Part model, mm, in its own coordinate system. A direction names the side the tool comes from. Round coordinates to 2 decimals unless told otherwise and drop trailing zeros. Loops run counter-clockwise (first coordinate to the right, second up) from the corner with the lowest first, then second, coordinate; pieces in that order, holes last.
(1) Probe probe 1 along X at (y, z) = (42, -6); probe 2 along Z at (x, y) = (13.5, 49); probe 3 along Y at (x, z) = (10, -10.5). List the from-to ranges inside material, lowest first.
(2) Cut at A-A on y = 47. List the corners of the cut face in (x, z), then the cut area to 3 significant figures.
(3) Tool access for faces 4 (the face through (0.57, 48.49, -0.6)), 5 (the face through (29.4, 48.49, -0.57)), 6 (the face through (15, 44, -25)), 7 (the face through (15, 48, 0)), 8 (the face through (15, 3, 14)): list every direction of +Z, -Z, +X, -X, +Y, -Y with a clear straight run to the whole face (end or side of a thin tool).
(4) Mould opens along X. For faces 1 (the face through (5, 44, -15)), 2 (the face through (0.6, 42.08, -29.43)), 3 (the face through (29.43, 42.08, -29.4)) say: +X half, -X half, draft (parallel to the pull), parting line (faces both ways), or undercut.
(5) Flat gauge pins, fed straight in: pin 1 (6 mm diameter, centred on x = 17.5, z = 28.5, fed in from -Y); pin 2 (6 mm diameter, centred on x = 11, y = 64, fed in from +Z); pin 3 (8 mm diameter, centred on x = 17.5, z = 14.5, fed in from +Y). Where does each tip first touch, or does it go through?
(6) Cut at D-D on y = 7.5. List the corners of the cut face in (x, z).
Autodesk Inventor part; units mm, degrees
ref_plane "YZ Plane" through (0, 0, 0) normal (1, 0, 0) x (0, 1, 0)
ref_plane "XZ Plane" through (0, 0, 0) normal (0, 1, 0) x (-1, 0, 0)
ref_plane "XY Plane" through (0, 0, 0) normal (0, 0, 1) x (1, 0, 0)
sketch "Sketch1" plane through (0, 0, 0) normal (1, 0, 0) x (0, 1, 0)
  line L0 (0, 0) -> (0, -30)
  line L1 (11, 0) -> (30, 0) construction
  line L2 (0, -30) -> (85, -30)
  line L3 (11, 0) -> (85, 0)
  line L4 (85, 0) -> (85, -30)
  line L5 (0, 0) -> (0, 14)
  line L6 (11, 0) -> (14, 0) construction
  line L7 (0, 14) -> (6, 14)
  line L8 (6, 14) -> (6, 34)
  line L9 (6, 34) -> (11, 34)
  line L10 (11, 34) -> (11, 0)
  dimension "d0" = 30
  dimension "d2" = 85
  dimension "d4" = 14
  dimension "d6" = 6
  dimension "d7" = 20
  dimension "d8" = 5
  dimension "d9" = 34
extrude "Extrusion1" add sketch "Sketch1" along normal blind 30
sketch "Sketch2" plane through (0, 85, 0) normal (0, 1, 0) x (1, 0, 0)
  line L0 (5, 5) -> (5, 25)
  line L1 (5, 5) -> (25, 5) construction
  line L2 (5, 25) -> (25, 25)
  line L3 (25, 25) -> (25, 5)
  line L4 (25, 5) -> (5, 5)
  point P0 (0, 0)
  dimension "d13" = 20
  dimension "d14" = 90
  dimension "d15" = 20
  dimension "d16" = 90
  dimension "d17" = 20
  dimension "d18" = 90
  dimension "d19" = 20
  dimension "d20" = 90
extrude "Extrusion2" cut sketch "Sketch2" against normal blind 80
fillet "Fillet1" radius 2 12 edges at (30, 85, -15) (15, 85, 0) (15, 85, -30) (0, 85, -15) (30, 48, 0) (30, 42.5, -30) (0, 48, 0) (0, 42.5, -30) (0, 11, 17) (15, 11, 34) (30, 11, 17) (15, 11, 0)
chamfer "Chamfer1" distance 3 angle 45 4 edges at (15, 85, -5) (5, 85, -15) (15, 85, -25) (25, 85, -15)
properties part number "flexibler_standfuß_v0.5"
Final values:
1. probe 1: x = 0 to 5, 25 to 30
1. probe 2: z = -30 to -25, -5 to 0
1. probe 3: y = 0 to 5
2. outline: (0, -28) arc R2 ccw to (2, -30) - (28, -30) arc R2 ccw to (30, -28) - (30, -2) arc R2 ccw to (28, 0) - (2, 0) arc R2 ccw to (0, -2) - close; hole (5, -25) - (25, -25) - (25, -5) - (5, -5) - close
2. area: 497 mm2
3. face 4: +Z, -X, +Y
3. face 5: +Z, +X, +Y
3. face 6: +Y
3. face 7: +Z, +X, -X, +Y
3. face 8: +Z, +X, -X, -Y
4. face 1: undercut
4. face 2: -X half
4. face 3: +X half
5. pin 1: stops at y = 6
5. pin 2: stops at z = 0
5. pin 3: stops at y = 11
6. outline: (0, -28) arc R2 ccw to (2, -30) - (28, -30) arc R2 ccw to (30, -28) - (30, 34) - (0, 34) - close; hole (5, -25) - (25, -25) - (25, -5) - (5, -5) - close
